Build history of the part. All positions in model axes, mm. A direction names the side the tool comes from. Round coordinates to 2 decimals unless told otherwise and drop trailing zeros. Loops run counter-clockwise (first coordinate to the right, second up) from the corner with the lowest first, then second, coordinate; pieces in that order, holes last. Notation, with made-up numbers: (67.5, 22.25) - (120.5, 22.25) arc R15 ccw to (120.5, 48.25) - close; hole circle Ø1 at (-16, 76.5). An arc over 180 degrees is marked (long way). Use one line per item in the form item = value. Start each with the question number.
Q1. Saw through at D-D (z = -6.75). Give the cut face in (x, y), then the cut area to 3 significant figures.
Q2. Mould opens along Y. For faces 1 (the face through (0.4, 28, -14)), 2 (the face through (-13.38, 25.73, -5.07)) say: released by +Y, released by -Y, zero draft, split by the parting line, or undercut.
Q3. Drill centre lines: line 1 (Y direction, x = 0, z = -6); line 2 (Y direction, x = 0, z = -0.3); line 3 (Y direction, x = -35, z = -0.05). Where is each one in solid material? Low to high.
Q4. Saw through at A-A (x = -35). Give the cut face in (y, z).
Q5. 3-axis set-ups, long thin cutter, end or side, ignore diameter. For faces 3 (the face through (-18.67, 19.07, -18.06)), 4 (the face through (-33.8, 0.9, -0.3)): which of +Z, -Z, +X, -X, +Y, -Y reach the whole face in a straight line?
Q6. Pin check, flat tips, straight feed: pin 1 (1.5 mm diameter, centred on x = 2, z = -2.5, fed in from +Y); pin 2 (5 mm diameter, centred on x = -16, z = -5.5, fed in from +Y); pin 3 (0.6 mm diameter, centred on x = 0, y = 29, fed in from -Z). Stop position of each tip, or through.
Q7. Saw through at C-C (z = -14.25). Give the cut face in (x, y).
```python
from build123d import *
from build123d.topology import SkipClean

# Parameters (mm, degrees)
CUT_EXTRUDE1_START = -10
CUT_EXTRUDE1_DEPTH = 10
SKETCH5_W          = 0.8
SKETCH5_H          = 8.001
CUT_EXTRUDE2_DEPTH = 57.722052077
CIRPATTERN1_COUNT  = 4


with BuildPart() as part:
    # Sketch1 → Revolve-Thin1 (revolve)
    with BuildSketch(Plane(origin=(0, 0, 0), x_dir=(0, 0, -1), z_dir=(1, 0, 0)), mode=Mode.PRIVATE) as revolve_thin1_sk:
        Polygon((0, 38), (0, 29), (10, 29), (18, 26.5), (18.149137497, 26.977239989), (10.076305461, 29.5), (0.5, 29.5), (0.5, 38), align=None)
    revolve(revolve_thin1_sk.sketch.rotate(Axis((0, 0, 0), (0, 0, 1)), 90), axis=Axis((0, 0, 0), (0, 0, 1)))

    # Sketch2 → Cut-Extrude1 (cut)
    with SkipClean():  # the faces are left unmerged after this step: merging them gives an invalid solid
        with BuildSketch(Plane(origin=(0, 0, -0.5), x_dir=(-1, 0, 0), z_dir=(0, 0, -1)).offset(CUT_EXTRUDE1_START)):
            with BuildLine():
                Line((-5, 37.669616404), (-5, 29.07318352))
                ThreePointArc((-5, 29.07318352), (-20.859650045, 20.859650045), (-29.07318352, 5))
                Line((-29.07318352, 5), (-37.669616404, 5))
                ThreePointArc((-37.669616404, 5), (-26.870057685, 26.870057685), (-5, 37.669616404))
            make_face()
        cut_extrude1 = extrude(amount=CUT_EXTRUDE1_DEPTH, mode=Mode.SUBTRACT)

    # Sketch3 → 3.0 _3_ Diameter Hole1 (revolve, cut)
    with SkipClean():  # the faces are left unmerged after this step: merging them gives an invalid solid
        with BuildSketch(Plane(origin=(0, 35, -0.5), x_dir=(0, 1, 0), z_dir=(1, 0, 0))):
            Polygon((0, 0), (0, 23.901290929), (1.5, 23), (1.5, 0), align=None)
        f_3_0_3_diameter_hole1 = revolve(axis=Axis((0, 35, -6.85), (0, 0, 1)), mode=Mode.SUBTRACT)

    # Sketch5 → Cut-Extrude2 (cut, through all)
    with SkipClean():  # the faces are left unmerged after this step: merging them gives an invalid solid
        with BuildSketch(Plane(origin=(0, 0, 0), x_dir=(1, 0, 0), z_dir=(0, 1, 0))):
            with Locations((0, 14.148637497)):
                Rectangle(SKETCH5_W, SKETCH5_H)
        cut_extrude2 = extrude(amount=-CUT_EXTRUDE2_DEPTH, mode=Mode.SUBTRACT)

    # CirPattern1: Cut-Extrude1, 3.0 _3_ Diameter Hole1, Cut-Extrude2 ×4 about axis
    with SkipClean():  # the faces are left unmerged after this step: merging them gives an invalid solid
        cirpattern1_axis = Axis((0, 0, 0), (0, 0, 1))
        add([cut_extrude1.rotate(cirpattern1_axis, i * 360 / CIRPATTERN1_COUNT) for i in range(1, CIRPATTERN1_COUNT)], mode=Mode.SUBTRACT)
        add([f_3_0_3_diameter_hole1.rotate(cirpattern1_axis, i * 360 / CIRPATTERN1_COUNT) for i in range(1, CIRPATTERN1_COUNT)], mode=Mode.SUBTRACT)
        add([cut_extrude2.rotate(cirpattern1_axis, i * 360 / CIRPATTERN1_COUNT) for i in range(1, CIRPATTERN1_COUNT)], mode=Mode.SUBTRACT)


solid = part.part
```
Report:
q1.outline = circle Ø59 at (0, 0); hole circle Ø58 at (0, 0)
q1.area = 91.9 mm²
q2.face_1 = zero draft
q2.face_2 = undercut
q3.line_1 = -29.5 to -29, 29 to 29.5
q3.line_2 = -38 to -36.5, -33.5 to -29, 29 to 33.5, 36.5 to 38
q3.line_3 = -5 to -1.5, 1.5 to 5
q4.outline = (-5, -0.5) - (-1.5, -0.5) - (-1.5, 0) - (-5, 0) - close; (1.5, -0.5) - (5, -0.5) - (5, 0) - (1.5, 0) - close
q5.face_3 = -Z
q5.face_4 = +Z, -Z
q6.pin_1 = 29.47
q6.pin_2 = 26.23
q6.pin_3 = -10.15
q7.outline = (-28.19, -0.4) arc R28.2 ccw to (-0.4, -28.19) - (-0.4, -27.67) arc R27.67 cw to (-27.67, -0.4) - close; (-28.19, 0.4) - (-27.67, 0.4) arc R27.67 cw to (-0.4, 27.67) - (-0.4, 28.19) arc R28.2 ccw to start; (0.4, -28.19) arc R28.2 ccw to (28.19, -0.4) - (27.67, -0.4) arc R27.67 cw to (0.4, -27.67) - close; (0.4, 27.67) arc R27.67 cw to (27.67, 0.4) - (28.19, 0.4) arc R28.2 ccw to (0.4, 28.19) - close
